Geometry check sheet. Reference: the model listing, model coordinates, mm. Face numbers are marked on the shaded views. Round coordinates to 2 decimals unless told otherwise and drop trailing zeros. Order: outer loops, then holes, each group sorted by start corner. A loop starts at its lowest first (then second) coordinate and runs counter-clockwise, first axis right, second up. Notation, with made-up numbers: (82, -39) -> (104, -39) arc R17 ccw to (104, -23) -> close; hole circle Ø5 at (-17.75, 62.25). An arc over 180 degrees is marked (long way). Use a Markdown table: item, result. Add a question column.
Item 1: Material ranges on probe 1 along Y at (x, z) = (17.5, -2); probe 2 along Y at (x, z) = (-6.5, 11); probe 3 along X at (y, z) = (17.5, 3.5), recorded low to high. Write a range as [from, to].
Item 2: Mould release check, pull along Y, two halves, no side actions. Record for the marked faces 1, 2 and 3: pulls with the +Y half, pulls with the -Y half, needs draft (parallel to the pull), parting line crosses it, or undercut.
Item 3: Gauge pin test, flat ends, axial feed: pin 1 Ø5 at (y, z) = (8, 12) entering from -X; pin 2 Ø12 at (x, y) = (-11.5, 12) entering from -Z; pin 3 Ø5 at (y, z) = (25, 15) entering from -X. Record the tip position at first contact, or that the pin passes through.
Item 4: Sectioned sample at A-A, the plane y = 22. Record the cut outline in (x, z).
Item 5: Sectioned sample at B-B, the plane y = 29. Record the cut outline in (x, z) (3 decimals), and give its area (3 significant figures).
from build123d import *

# Parameters (mm, degrees)
FILLET1_R = 5
FILLET2_R = 0.5
FILLET3_R = 0.5


with BuildPart() as part:
    # Sketch1 → Revolve1 (revolve)
    with BuildSketch(Plane(origin=(0, 0, 0), x_dir=(0, 0, -1), z_dir=(1, 0, 0))):
        Polygon((20, 0), (0, 0), (0, 32), (20, 32), (10, 16), align=None)
        Polygon((18.125, 3), (20, 0), (20, 3), align=None)
    revolve(axis=Axis((0, 0, 0), (0, 1, 0)))

    # Fillet1
    fillet1_edges = [part.edges().sort_by_distance(p)[0] for p in [
        (0, 16, 10),
    ]]
    fillet(fillet1_edges, radius=FILLET1_R)

    # Fillet2
    fillet2_edges = [part.edges().sort_by_distance(p)[0] for p in [
        (0, 32, 20),
    ]]
    fillet(fillet2_edges, radius=FILLET2_R)

    # Fillet3
    fillet3_edges = [part.edges().sort_by_distance(p)[0] for p in [
        (0, 3, 20),
    ]]
    fillet(fillet3_edges, radius=FILLET3_R)


solid = part.part
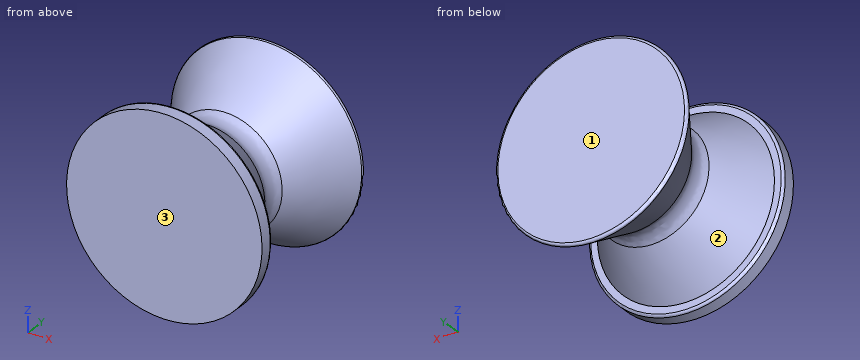
Found:
| question | item | result |
|---|---|---|
| 1 | probe 1 | y = [0, 3.82], [28.18, 32] |
| 1 | probe 2 | y = [0, 11.56], [20.44, 32] |
| 1 | probe 3 | x = [-10.56, 10.56] |
| 2 | face 1 | pulls with the +Y half |
| 2 | face 2 | undercut |
| 2 | face 3 | pulls with the -Y half |
| 3 | pin 1 | stops at x = -12.44 |
| 3 | pin 2 | stops at z = -13.34 |
| 3 | pin 3 | stops at x = -10.26 |
| 4 | outline | circle Ø27.5 at (0, 0) |
| 5 | outline | circle Ø36.25 at (0, 0) |
| 5 | area | 1,030 mm2 |
